Build history of the part. All positions in model axes, mm. Face numbers are marked on the shaded views. A direction names the side the tool comes from. Round coordinates to 2 decimals unless told otherwise and drop trailing zeros. Loops run counter-clockwise (first coordinate to the right, second up) from the corner with the lowest first, then second, coordinate; pieces in that order, holes last. Notation, with made-up numbers: (22, 45) - (57, 45) arc R15 cw to (57, 70) - close; hole circle Ø8 at (77.25, 20.5). An arc over 180 degrees is marked (long way). Use a Markdown table: item, result.
from build123d import *

# Parameters (mm, degrees)
BOSS_EXTRUDE1_DEPTH = 20
SCALE1_SCALE        = 0.110510806
SKETCH5_R           = 2.4
BOSS_EXTRUDE2_DEPTH = 10


with BuildPart() as part:
    # Sketch3 → Boss-Extrude1 (new body)
    with BuildSketch(Plane(origin=(0, 0, 0), x_dir=(0, 0, -1), z_dir=(1, 0, 0))):
        with BuildLine():
            Line((0, -60), (0, -86.184781703))
            ThreePointArc((0, -86.184781703), (14.644660941, -121.540120762), (50, -136.184781703))
            Line((50, -136.184781703), (59.297038535, -136.184781703))
            Line((59.297038535, -136.184781703), (138.939006392, -136.184781703))
            ThreePointArc((138.939006392, -136.184781703), (153.081142016, -130.326917326), (158.939006392, -116.184781703))
            Line((158.939006392, -116.184781703), (158.939006392, -50))
            Line((158.939006392, -50), (158.939006392, -11.480346054))
            ThreePointArc((158.939006392, -11.480346054), (148.053108697, 21.328755123), (117.156078712, 36.830801017))
            ThreePointArc((117.156078712, 36.830801017), (39.60735059, 11.368133348), (0, -60))
        make_face()
    extrude(amount=BOSS_EXTRUDE1_DEPTH)


with BuildPart() as part_1:
    # Scale1: scaled about (10, -55.771836123, -85.371281571)
    add(part.part.scale(SCALE1_SCALE).moved(Location((8.89489194, -49.608445561, -75.936832435))))

    # Sketch5 → Boss-Extrude2 (add)
    with BuildSketch(Plane.ZY.offset(-8.89489194)):
        with Locations((-85.501310137, -55.288244055)):
            Circle(SKETCH5_R)
    extrude(amount=BOSS_EXTRUDE2_DEPTH)


solid = part_1.part
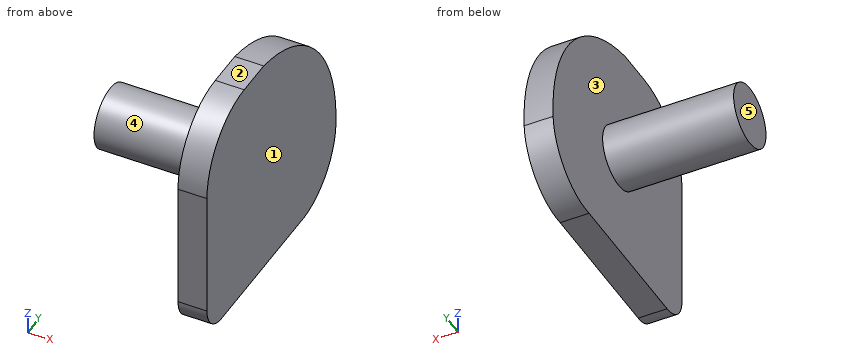
Q1. Which spindle directions (+Z, -Z, +X, -X, +Y, -Y) get a long thin tool onto all of the face, cutting with end or side? Do the marked faces 4 and 5. Say none if no direction does.
Results found:
| item | result |
|---|---|
| face 4 | -X |
| face 5 | +Z, -Z, -X, +Y, -Y |
Q2. Pull direction X, two halves, no side cores. Call the marked faces 1, 2 and 3: pulls with the +X half, pulls with the -X half, needs draft (parallel to the pull), parting line crosses it, or undercut.
Results found:
| item | result |
|---|---|
| face 1 | pulls with the +X half |
| face 2 | needs draft |
| face 3 | pulls with the -X half |
Q3. Probe line 1 (X direction, y = -48.25, z = -87.75); line 2 (Z direction, x = 2.75, y = -55.25); line 3 (Y direction, x = 1.25, z = -87.5). List the from-to ranges inside material, lowest first.
Results found:
| item | result |
|---|---|
| line 1 | x = 8.89 to 11.11 |
| line 2 | z = -87.9 to -83.1 |
| line 3 | y = -56.62 to -53.96 |
Q4. Drop flat-ended pins along their axis: pin 1 (1 mm diameter, centred on x = 6.5, z = -85.5, fed in from -Y); pin 2 (1.1 mm diameter, centred on x = 9.5, y = -57, fed in from -Z); pin 3 (4 mm diameter, centred on x = 5.5, y = -48, fed in from -Z); pin 4 (1 mm diameter, centred on x = 5.5, y = -56.5, fed in from -Z). Give the stop position or say it passes through.
Results found:
| item | result |
|---|---|
| pin 1 | stops at y = -57.69 |
| pin 2 | stops at z = -93.5 |
| pin 3 | passes through |
| pin 4 | stops at z = -87.79 |
Q5. Cut at A-A, the plane y = -58.5. List the corners of the cut face in (x, z).
Results found:
| item | result |
|---|---|
| outline | (8.89, -93.5) - (11.11, -93.5) - (11.11, -75.94) - (8.89, -75.94) - close |
Q6. Cut at D-D, the plane y = -55. List the corners of the cut face in (x, z).
Results found:
| item | result |
|---|---|
| outline | (-1.11, -87.88) - (8.89, -87.88) - (8.89, -93.5) - (11.11, -93.5) - (11.11, -76.17) - (8.89, -76.17) - (8.89, -83.12) - (-1.11, -83.12) - close |
Q7. Cut at C-C, the plane x = 1.5. List the corners of the cut face in (y, z), plus the area to 3 significant figures.
Results found:
| item | result |
|---|---|
| outline | circle Ø4.8 at (-55.29, -85.5) |
| area | 18.1 mm2 |
Q8. Cut at B-B, the plane z = -84. List the corners of the cut face in (x, y).
Results found:
| item | result |
|---|---|
| outline | (-1.11, -57.16) - (8.89, -57.16) - (8.89, -64.66) - (11.11, -64.66) - (11.11, -46.25) - (8.89, -46.25) - (8.89, -53.42) - (-1.11, -53.42) - close |
